Read the model definition and answer for the solid it produces. Units are mm, in the model's axes. A direction names the side the tool comes from. Give positions to 0.01 mm unless a question says otherwise; leave off trailing zeros. Loops run counter-clockwise (first coordinate to the right, second up) from the corner with the lowest first, then second, coordinate; pieces in that order, holes last. Notation, with made-up numbers: (-3, -12) - (18, -12) arc R23 ccw to (18, 15) - close; hole circle Ø1 at (18, 63). An arc over 180 degrees is marked (long way). Put each result on its own line as item: value. Start each with the question number.
1. For a pull along Z with two mould halves and no side action, classify faces 1 (the cylindrical face through (1.542, 2.839, 5.896)), 2 (the cylindrical face through (-5.37, 0.48, -1.19)), 3 (the flat face through (-1.3, 2.3, 1.3)) as released by +Z, released by -Z, zero draft, split by the parting line, or undercut.
2. A cutting plane is placed at D-D, the plane z = 12. Determine the outline of the cut face in (x, y), plus the area to 3 significant figures.
3. A cutting plane is placed at A-A, the plane y = 4. Determine the outline of the cut face in (x, z) (3 decimals).
4. A cutting plane is placed at B-B, the plane x = 11.5. Determine the outline of the cut face in (y, z), plus the area to 3 significant figures.
5. Given pin 1 Ø5 at (x, z) = (11, -2) entering from +Y; pin 2 Ø4 at (y, z) = (0.5, 6.5) entering from -X; pin 3 Ø5 at (x, z) = (11.5, 4.5) entering from -Y; pin 4 Ø5 at (x, z) = (0, 0) entering from -Y, each flat-ended and moving along its own axis, determine where each tip first touches the part or whether it passes through.
6. For faces 4 (the flat face through (11.789, 2.761, 8.654)), 5 (the cylindrical face through (0.9, 3.97, 2.86)), 6 (the flat face through (8, 5.6, 3)), determine the directions among +Z, -Z, +X, -X, +Y, -Y from which every point of the face is accessible in a straight line to the end or side of a thin tool.
7. A cutting plane is placed at C-C, the plane z = 5.05. Determine the outline of the cut face in (x, y).
8. Consider L1, parallel to Z at x = 9.75, y = 2.75; L2, parallel to Z at x = 13, y = 1.75; L3, parallel to Y at x = 19, z = 11.5. Determine where each line is inside the solid, lowest interval first. Write a range as from..to.
```python
from build123d import *

# Parameters (mm, degrees)
EXTRUDE_THIN2_DEPTH = 5.6
BOSS_EXTRUDE1_DEPTH = 5.6
BOSS_EXTRUDE2_START = -4.5
SKETCH6_R           = 5.5
BOSS_EXTRUDE2_DEPTH = 10.1
FILLET1_R           = 10
SKETCH7_R           = 2.59
CUT_EXTRUDE3_DEPTH  = 4
CUT_EXTRUDE4_DEPTH  = 4
CIRPATTERN1_COUNT   = 25
SKETCH9_R           = 3
CUT_EXTRUDE5_DEPTH  = 3.3
SKETCH10_R          = 1.6
CUT_EXTRUDE6_DEPTH  = 26.423002314


with BuildPart() as part:
    # Sketch4 → Extrude-Thin2 (new body)
    with BuildSketch(Plane(origin=(0, 0, 0), x_dir=(1, 0, 0), z_dir=(0, 1, 0))):
        with BuildLine():
            Line((10.796856578, -1.499295844), (18.374578861, -5.874295844))
            ThreePointArc((18.374578861, -5.874295844), (19.875283017, -11.475), (14.274578861, -12.975704156))
            Line((14.274578861, -12.975704156), (6.696856578, -8.600704156))
            ThreePointArc((6.696856578, -8.600704156), (5.196152423, -3), (10.796856578, -1.499295844))
        make_face()
        with BuildLine():
            Line((9.546856578, -3.664359354), (17.124578861, -8.039359354))
            ThreePointArc((17.124578861, -8.039359354), (17.710219507, -10.225), (15.524578861, -10.810640646))
            Line((15.524578861, -10.810640646), (7.946856578, -6.435640646))
            ThreePointArc((7.946856578, -6.435640646), (7.361215932, -4.25), (9.546856578, -3.664359354))
        make_face(mode=Mode.SUBTRACT)
    extrude(amount=EXTRUDE_THIN2_DEPTH)

    # Sketch5 → Boss-Extrude1 (add)
    with BuildSketch(Plane(origin=(0, 0, 0), x_dir=(1, 0, 0), z_dir=(0, 1, 0))):
        with BuildLine():
            Line((10.796856578, -1.499295844), (2.05, 3.550704156))
            ThreePointArc((2.05, 3.550704156), (-3.550704156, 2.05), (-2.05, -3.550704156))
            Line((-2.05, -3.550704156), (6.696856578, -8.600704156))
            ThreePointArc((6.696856578, -8.600704156), (8.998238507, -9.142286296), (11.216030786, -8.323099255))
            Line((11.216030786, -8.323099255), (7.946856578, -6.435640646))
            ThreePointArc((7.946856578, -6.435640646), (7.361215932, -4.25), (9.546856578, -3.664359354))
            Line((9.546856578, -3.664359354), (12.816030786, -5.551817963))
            ThreePointArc((12.816030786, -5.551817963), (12.416571434, -3.221559989), (10.796856578, -1.499295844))
        make_face()
    extrude(amount=BOSS_EXTRUDE1_DEPTH)

    # Sketch6 → Boss-Extrude2 (add)
    with BuildSketch(Plane(origin=(0, 0, 0), x_dir=(1, 0, 0), z_dir=(0, 1, 0)).offset(BOSS_EXTRUDE2_START)):
        with Locations(Location((0, 0, 0), (0, 0, 270))):
            Circle(SKETCH6_R)
    extrude(amount=BOSS_EXTRUDE2_DEPTH)

    # Fillet1
    # the kernel refuses this fillet: 10 mm, written as the material it adds along each edge
    with BuildSketch(Plane(origin=(1.124901573, 5.6, 5.383734433), x_dir=(-0.998469356889102, 0, 0.05530771513507689), z_dir=(0, -1, 0))) as fillet1_piece_1:
        with BuildLine():
            CenterArc((3.151594855, -9.886744715), FILLET1_R, 98.631327733, 24.539188727)
            Line((-2.319730793, -1.516285011), (0, 0))
            ThreePointArc((0, 0), (0.8254177, -0.062290407), (1.6508354, 0))
        make_face()
    extrude(amount=5.6)
    with BuildSketch(Plane(origin=(5.224901573, 5.6, -1.717673878), x_dir=(0.8660254037844397, 0, 0.49999999999999806), z_dir=(0, -1, 0))) as fillet1_piece_2:
        with BuildLine():
            CenterArc((2.77133022, -10), FILLET1_R, 90, 24.539188727)
            ThreePointArc((-1.381825119, -0.903225806), (-0.65683145, -0.503752837), (0, 0))
            Line((0, 0), (2.77133022, 0))
        make_face()
    extrude(amount=5.6)

    # Sketch7 → Cut-Extrude3 (cut)
    with BuildSketch(Plane.XZ.offset(4.5)):
        with Locations(Location((0, 0, 0), (0, 0, 270))):
            Circle(SKETCH7_R)
    extrude(amount=-CUT_EXTRUDE3_DEPTH, mode=Mode.SUBTRACT)

    # Sketch8 → Cut-Extrude4 (cut)
    with BuildSketch(Plane.XZ.offset(4.5)):
        with BuildLine():
            Line((0, 3.04), (0, 2.59))
            ThreePointArc((0, 2.59), (0.162627446, 2.584889227), (0.324613075, 2.569577076))
            Line((0.324613075, 2.569577076), (0.15, 3.04))
            Line((0.15, 3.04), (0, 3.04))
        make_face()
        with BuildLine():
            ThreePointArc((-0.324613075, 2.569577076), (-0.162627446, 2.584889227), (0, 2.59))
            Line((0, 2.59), (0, 3.04))
            Line((0, 3.04), (-0.15, 3.04))
            Line((-0.15, 3.04), (-0.324613075, 2.569577076))
        make_face()
    cut_extrude4 = extrude(amount=-CUT_EXTRUDE4_DEPTH, mode=Mode.SUBTRACT)

    # CirPattern1: Cut-Extrude4 ×25 about axis
    cirpattern1_axis = Axis((0, 0, 0), (0, 1, 0))
    for i in range(1, CIRPATTERN1_COUNT):
        add(cut_extrude4.rotate(cirpattern1_axis, i * 360 / CIRPATTERN1_COUNT), mode=Mode.SUBTRACT)

    # Sketch9 → Cut-Extrude5 (cut)
    with BuildSketch(Plane(origin=(0, 5.6, 0), x_dir=(1, 0, 0), z_dir=(0, 1, 0))):
        with Locations(Location((0, 0, 0), (0, 0, 270))):
            Circle(SKETCH9_R)
    extrude(amount=-CUT_EXTRUDE5_DEPTH, mode=Mode.SUBTRACT)

    # Sketch10 → Cut-Extrude6 (cut, through all)
    with BuildSketch(Plane(origin=(0, 2.3, 0), x_dir=(1, 0, 0), z_dir=(0, 1, 0))):
        with Locations(Location((0, 0, 0), (0, 0, 270))):
            Circle(SKETCH10_R)
    extrude(amount=-CUT_EXTRUDE6_DEPTH, mode=Mode.SUBTRACT)


solid = part.part
```
Return value:
1. face 1: released by +Z
1. face 2: split by the parting line
1. face 3: undercut
2. outline: (12.58, 0) - (19.52, 0) - (19.52, 5.6) - (12.58, 5.6) - close
2. area: 38.8 mm2
3. outline: (-0.523, 5.475) arc R5.5 ccw (long way) to (4.48, -3.191) arc R10 cw to (7.625, -0.332) - (18.375, 5.874) arc R4.1 ccw to (14.275, 12.976) - (3.525, 6.769) arc R10 cw to start; hole circle Ø6 at (0, 0); hole (7.947, 6.436) arc R1.6 ccw to (9.547, 3.664) - (17.125, 8.039) arc R1.6 ccw to (15.525, 10.811) - close
4. outline: (0, 1.91) - (5.6, 1.91) - (5.6, 4.79) - (0, 4.79) - close; (0, 8.49) - (5.6, 8.49) - (5.6, 11.37) - (0, 11.37) - close
4. area: 32.3 mm2
5. pin 1: passes through
5. pin 2: stops at x = -3.16
5. pin 3: stops at y = 0
5. pin 4: stops at y = -0.5
6. face 4: +Y, -Y
6. face 5: +Y
6. face 6: +Z, -Z, +X, -X, +Y
7. outline: (-2.18, -4.5) - (2.18, -4.5) - (2.18, 0) - (7.15, 0) - (7.15, 5.6) - (-2.18, 5.6) - close; (11.95, 0) - (16.95, 0) - (16.95, 5.6) - (11.95, 5.6) - close
8. L1: z = 0.89..3.78, 7.48..10.36
8. L2: z = 2.77..5.66, 9.35..12.24
8. L3: y = 0..5.6
